Source: three-view drawing plus pictorial views. Frame: mm from the lowest corner of the part. Give positions to 0.01 mm unless a question says otherwise; leave off trailing zeros. Order: outer loops, then holes, each group sorted by start corner. A loop starts at its lowest first (then second) coordinate and runs counter-clockwise, first axis right, second up. Notation, with made-up numbers: (7.5, 28.25) -> (17.5, 28.25) arc R22 ccw to (17.5, 38.25) -> close; hole circle Ø2 at (38, -1). An arc over 180 degrees is marked (long way). Answer in a Markdown table with one row per item. Add a question column.
Q1. Line query: line 1 along Y through (x, z) = (14, 2.2); line 2 along Y through (x, z) = (13, 3.3); line 3 along X through (y, z) = (28.5, 3.05). Output: solid intervals per line, ascending. Write a range as from..to.
Q2. Cut plane A-A on y = 75. Return the cut outline in (x, z).
Q3. Cut plane B-B on x = 14. Return the cut outline in (y, z), and give its area (3 significant figures).
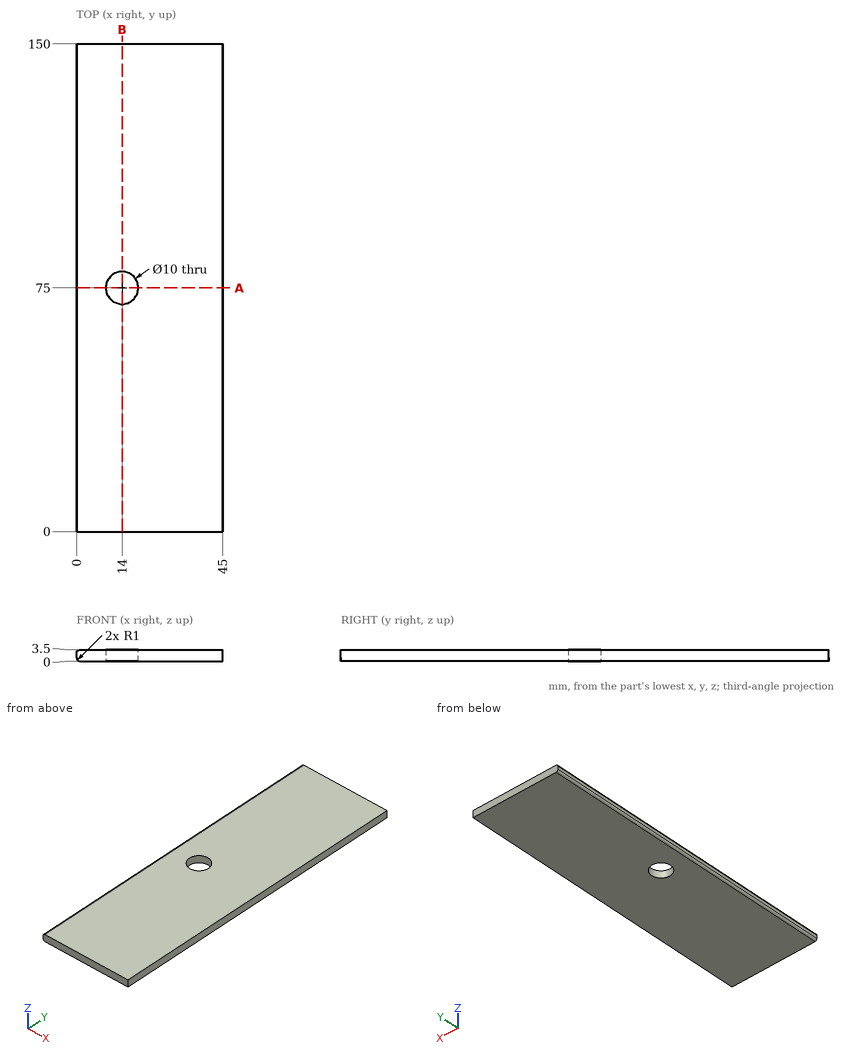
Completed:
| question | item | result |
|---|---|---|
| 1 | line 1 | y = 0..70, 80..150 |
| 1 | line 2 | y = 0..70.1, 79.9..150 |
| 1 | line 3 | x = 0.16..45 |
| 2 | outline | (0, 1) arc R1 ccw to (1, 0) -> (9, 0) -> (9, 3.5) -> (1, 3.5) arc R1 ccw to (0, 2.5) -> close; (19, 0) -> (45, 0) -> (45, 3.5) -> (19, 3.5) -> close |
| 3 | outline | (0, 0) -> (70, 0) -> (70, 3.5) -> (0, 3.5) -> close; (80, 0) -> (150, 0) -> (150, 3.5) -> (80, 3.5) -> close |
| 3 | area | 490 mm² |
